Source: CAD feature listing. Evaluate the final solid. Frame: model axes, mm. Face numbers are marked on the shaded views. Coordinates: 2 decimals unless noted, no trailing zeros. Write each loop counter-clockwise with the first axis right and the second up, starting at its lowest first coordinate (ties: lowest second). Pieces come first, ordered by that corner, then holes. Notation, with made-up numbers: (16.25, -6) -> (30.25, -6) arc R15 ccw to (30.25, 18) -> close; hole circle Ø8 at (35.25, -13.5). An arc over 180 degrees is marked (long way). Write item = value, one per line.
from build123d import *

# Parameters (mm, degrees)
SKETCH1_R                       = 41.91
SKETCH1_R_2                     = 39.624
BOSS_EXTRUDE2_DEPTH             = 12.7
SKETCH2_R                       = 2.54
CUT_EXTRUDE1_DEPTH              = 56.7
CIRPATTERN1_COUNT               = 8
CIRPATTERN2_COUNT               = 2
CIRPATTERN2_ANGLE               = 70
CIRPATTERN2_THE_OTHER_WAY_COUNT = 2
CIRPATTERN2_THE_OTHER_WAY_ANGLE = 70


with BuildPart() as part:
    # Sketch1 → Boss-Extrude2 (new body)
    with BuildSketch(Plane(origin=(0, 0, 0), x_dir=(1, 0, 0), z_dir=(0, 1, 0))):
        with Locations(Location((0, 0, 0), (0, 0, 270))):
            Circle(SKETCH1_R)
        with Locations(Location((0, 0, 0), (0, 0, 270))):
            Circle(SKETCH1_R_2, mode=Mode.SUBTRACT)
    extrude(amount=BOSS_EXTRUDE2_DEPTH)

    # Sketch2 → Cut-Extrude1 (cut)
    with BuildSketch(Plane.XY):
        with Locations(Location((0, 6.35, 0), (0, 0, 90))):
            Circle(SKETCH2_R)
    cut_extrude1 = extrude(amount=-CUT_EXTRUDE1_DEPTH, mode=Mode.SUBTRACT)

    # CirPattern1: Cut-Extrude1 ×8 about axis
    cirpattern1_axis = Axis((0, 12.7, 0), (0, 1, 0))
    for i in range(1, CIRPATTERN1_COUNT):
        add(cut_extrude1.rotate(cirpattern1_axis, i * 360 / CIRPATTERN1_COUNT), mode=Mode.SUBTRACT)

    # CirPattern2: Cut-Extrude1 ×2 about axis
    cirpattern2_axis = Axis((0, 12.7, 0), (0, 1, 0))
    for i in range(1, CIRPATTERN2_COUNT):
        add(cut_extrude1.rotate(cirpattern2_axis, i * CIRPATTERN2_ANGLE / (CIRPATTERN2_COUNT - 1)), mode=Mode.SUBTRACT)

    # CirPattern2 the other way: Cut-Extrude1 ×2 about axis
    cirpattern2_the_other_way_axis = Axis((0, 12.7, 0), (0, -1, 0))
    for i in range(1, CIRPATTERN2_THE_OTHER_WAY_COUNT):
        add(cut_extrude1.rotate(cirpattern2_the_other_way_axis, i * CIRPATTERN2_THE_OTHER_WAY_ANGLE / (CIRPATTERN2_THE_OTHER_WAY_COUNT - 1)), mode=Mode.SUBTRACT)


solid = part.part
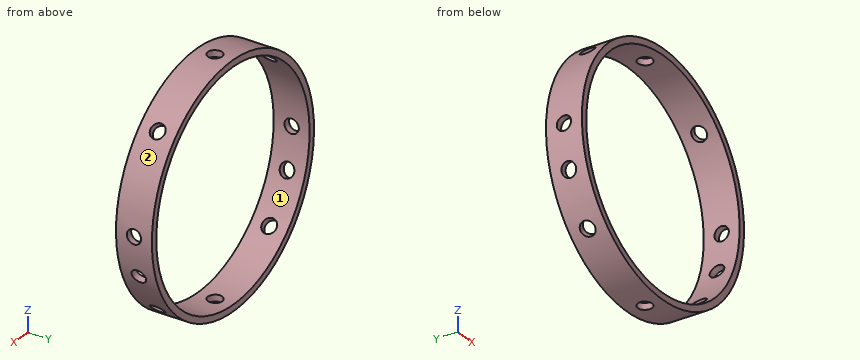
1) Cut plane A-A, the plane z = 0. Output: boundary loops of the cut face in (x, y), and give its area (3 significant figures).
Answer block:
outline = (-41.91, 0) -> (-39.62, 0) -> (-39.62, 3.81) -> (-41.91, 3.81) -> close; (-41.91, 8.89) -> (-39.62, 8.89) -> (-39.62, 12.7) -> (-41.91, 12.7) -> close; (39.62, 0) -> (41.91, 0) -> (41.91, 3.81) -> (39.62, 3.81) -> close; (39.62, 8.89) -> (41.91, 8.89) -> (41.91, 12.7) -> (39.62, 12.7) -> close
area = 34.8 mm2
2) Cut plane D-D, the plane y = 10. Output: boundary loops of the cut face in (x, z).
Answer block:
outline = circle Ø83.82 at (0, 0); hole circle Ø79.25 at (0, 0)
3) Pull-direction query (X, two-part tool) for the marked faces 1 and 2; classes: +X half, -X half, draft (parallel to the pull), parting line (faces both ways), or undercut.
Answer block:
face_1 = undercut
face_2 = parting line
4) First-contact query: pin 1 Ø6 at (y, z) = (4.5, 24.5) entering from +X; pin 2 Ø2 at (y, z) = (10, 25) entering from -X; pin 3 Ø4 at (x, y) = (19, 8.5) entering from +Z. Flat tips, straight axial feed; report the tip coordinate or a pass-through.
Answer block:
pin_1 = 35.97
pin_2 = -34.36
pin_3 = 38.31
5) Cut plane C-C, the plane z = 24.5. Output: boundary loops of the cut face in (x, y).
Answer block:
outline = (-34, 0) -> (-31.14, 0) -> (-31.14, 12.7) -> (-34, 12.7) -> close; (31.14, 0) -> (34, 0) -> (34, 12.7) -> (31.14, 12.7) -> close
6) Material intervals for probe 1 along Y at (x, z) = (-41.1, 0); probe 2 along X at (y, z) = (12, 1); probe 3 along X at (y, z) = (8, 23.5), sorted ascending. Write a range as [from, to].
Answer block:
probe_1 = [0, 3.81], [8.89, 12.7]
probe_2 = [-41.9, -39.61], [39.61, 41.9]
probe_3 = [-34.7, -31.9], [31.9, 34.7]
7) Cut plane B-B, the plane x = -11. Output: boundary loops of the cut face in (y, z), and give its area (3 significant figures).
Answer block:
outline = (0, -40.44) -> (12.7, -40.44) -> (12.7, -38.07) -> (0, -38.07) -> close; (0, 38.07) -> (12.7, 38.07) -> (12.7, 40.44) -> (0, 40.44) -> close
area = 60.3 mm2
